from build123d import *

# Parameters (mm, degrees)
F0_W     = 120
F0_H     = 150
F1_DEPTH = 56
F3_DEPTH = 67.5


with BuildPart() as f1:
    # F0 (on Top) → F1 (new body)
    with BuildSketch(Plane.XY):
        Rectangle(F0_W, F0_H)
    extrude(amount=F1_DEPTH)

    # F2 (on face) → F3 (cut)
    with BuildSketch(Plane.XY.offset(56)):
        with BuildLine():
            Line((-54, 65.75), (-54, 69))
            Line((-54, 69), (-50.75, 69))
            ThreePointArc((-50.75, 69), (-56.298097, 71.298097), (-54, 65.75))
        make_face()
        with BuildLine():
            Line((-50.75, 69), (-54, 69))
            Line((-54, 69), (-54, 65.75))
            ThreePointArc((-54, 65.75), (-51.701903, 66.701903), (-50.75, 69))
        make_face()
        with BuildLine():
            ThreePointArc((57.25, 69), (54, 72.25), (50.75, 69))
            Line((50.75, 69), (54, 69))
            Line((54, 69), (54, 65.75))
            ThreePointArc((54, 65.75), (56.298097, 66.701903), (57.25, 69))
        make_face()
        with BuildLine():
            Line((54, 69), (50.75, 69))
            ThreePointArc((50.75, 69), (51.701903, 66.701903), (54, 65.75))
            Line((54, 65.75), (54, 69))
        make_face()
        with BuildLine():
            Line((-54, -69), (-54, -65.75))
            ThreePointArc((-54, -65.75), (-56.298097, -71.298097), (-50.75, -69))
            Line((-50.75, -69), (-54, -69))
        make_face()
        with BuildLine():
            ThreePointArc((-50.75, -69), (-51.701903, -66.701903), (-54, -65.75))
            Line((-54, -65.75), (-54, -69))
            Line((-54, -69), (-50.75, -69))
        make_face()
        with BuildLine():
            ThreePointArc((57.25, -69), (56.298097, -66.701903), (54, -65.75))
            Line((54, -65.75), (54, -69))
            Line((54, -69), (50.75, -69))
            ThreePointArc((50.75, -69), (54, -72.25), (57.25, -69))
        make_face()
        with BuildLine():
            Line((54, -69), (54, -65.75))
            ThreePointArc((54, -65.75), (51.701903, -66.701903), (50.75, -69))
            Line((50.75, -69), (54, -69))
        make_face()
    extrude(amount=-F3_DEPTH, mode=Mode.SUBTRACT)


solid = f1.part
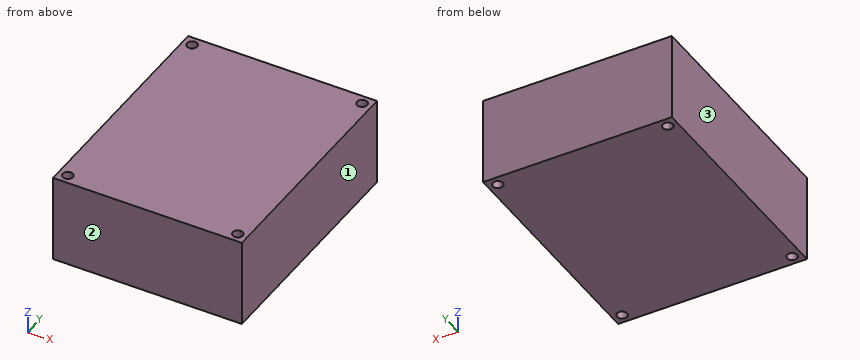
Read the model definition and answer for the solid it produces. Units are mm, in the model's axes. Face numbers are marked on the shaded views. Give positions to 0.01 mm unless a question says otherwise; leave off trailing zeros. One line per item, written item: value. Start each with the question number.
(1) Find the intervals of material crossed by line 1 (Y direction, x = -54, z = 29); line 2 (X direction, y = -69, z = 22.5); line 3 (X direction, y = 66, z = 17.5), in increasing order.
(2) A flat-ended cylindrical pin translates along its axis: pin 1 Ø5 at (x, y) = (-54, -69) entering from -Z. Find the tip coordinate at first contact, or state that the pin passes through.
(3) Determine the mould class of the marked faces 1, 2 and 3 for opening direction X: pulls with the +X half, pulls with the -X half, needs draft (parallel to the pull), parting line crosses it, or undercut.
Results below:
1. line 1: y = -75 to -72.25, -65.75 to 65.75, 72.25 to 75
1. line 2: x = -60 to -57.25, -50.75 to 50.75, 57.25 to 60
1. line 3: x = -60 to -55.25, -52.75 to 52.75, 55.25 to 60
2. pin 1: passes through
3. face 1: pulls with the +X half
3. face 2: needs draft
3. face 3: pulls with the -X half
